Check sheet for the modelled part. Datum: model origin and axes. Units: mm. Face numbers are marked on the shaded views. A direction names the side the tool comes from. Round coordinates to 2 decimals unless told otherwise and drop trailing zeros. Loops run counter-clockwise (first coordinate to the right, second up) from the corner with the lowest first, then second, coordinate; pieces in that order, holes last. Notation, with made-up numbers: M 37.25,40.25 L 75.25,40.25 A18 cw 75.25,64.25 Z; hole C -12.75,-40 d1. An arc over 180 degrees is marked long. Write item = value, one per line. Start each with the question number.
(1) Cross-section at A-A on z = 7. Record the boundary of the cut face in (x, y), plus the area to 3 significant figures.
(2) Scan lines: L1, parallel to Y at x = 0, z = 14.6; L2, parallel to Y at x = 0, z = 10.7; L3, parallel to X at y = 12.5, z = 10.95. Record each from-to range of solid material in increasing order. Write a range as from..to.
(3) Set-up check for the marked faces 1 and 2: record each of +Z, -Z, +X, -X, +Y, -Y from which the full face is reachable in a straight line by a thin tool's end or side.
(4) Mould release check, pull along X, two halves, no side actions. Record for the marked faces 3, 4 and 5: pulls with the +X half, pulls with the -X half, needs draft (parallel to the pull), parting line crosses it, or undercut.
(5) Go/stop test with flat-tipped pins: P1, Ø2, axis at y = 19.5, z = 2.5, coming from the -X side; P2, Ø4, axis at x = 7.5, z = 5.5, coming from the -Y side; P3, Ø1, axis at x = -21, y = 13, coming from the -Z side. Record where each tip stops, or that it passes through.
(6) Cross-section at B-B on x = -11. Record the boundary of the cut face in (y, z).
(7) Cross-section at C-C on y = 5.5. Record the boundary of the cut face in (x, z).
Autodesk Fusion 360 part; units mm, degrees
sketch "Sketch1" plane through (0, 0, 0) normal (0, 0, 1) x (1, 0, 0)
  circle A0 centre (0, 0) radius 30 construction
  circle A1 centre (0, 0) radius 32
  circle A2 centre (0, 0) radius 34
  dimension "d10" = 60
  dimension "d11" = 2
  dimension "d12" = 4
extrude "Extrude1" add sketch "Sketch1" along normal blind 16.6 contours A1 | A2
extrude "Extrude2" cut sketch "Sketch1" along normal blind 12.6 contours A1
sketch "Sketch2" plane through (0, 0, 16.6) normal (0, 0, 1) x (-1, 0, 0)
  circle A0 centre (0, 0) radius 34
  circle A1 centre (0, 0) radius 2.75
  line L0 (0, 0) -> (0, 15) construction
  circle A2 centre (0, 15) radius 3.65
  line L1 (0, 0) -> (-13.0112, 31.4119) construction
  line L2 (0, 0) -> (34, 0) construction
  line L3 (0.4619, 0.1913) -> (-12.5493, 31.6032)
  line L4 (-0.4619, -0.1913) -> (-13.4732, 31.2206)
  line L5 (0.5729, 2.6897) -> (12.5493, 31.6032)
  line L6 (1.4968, 2.307) -> (13.4732, 31.2206)
  line L7 (2.307, 1.4968) -> (31.2206, 13.4732)
  line L8 (2.6897, 0.5729) -> (31.6032, 12.5493)
  line L9 (2.6897, -0.5729) -> (31.6032, -12.5493)
  line L10 (2.307, -1.4968) -> (31.2206, -13.4732)
  line L11 (1.4968, -2.307) -> (13.4732, -31.2206)
  line L12 (0.5729, -2.6897) -> (12.5493, -31.6032)
  line L13 (-0.5729, -2.6897) -> (-12.5493, -31.6032)
  line L14 (-1.4968, -2.307) -> (-13.4732, -31.2206)
  line L15 (-2.307, -1.4968) -> (-31.2206, -13.4732)
  line L16 (-2.6897, -0.5729) -> (-31.6032, -12.5493)
  line L17 (-2.6897, 0.5729) -> (-31.6032, 12.5493)
  line L18 (-2.307, 1.4968) -> (-31.2206, 13.4732)
  circle A3 centre (0, 15) radius 3.15
  line L19 (3.1499, 14.9727) -> (3.1339, 13.1289)
  line L20 (-3.15, 15) -> (-3.15, 13.1561)
  dimension "d35" = 5.5
  dimension "d38" = 15
  dimension "d39" = 7.3
  dimension "d42" = 112.5
  dimension "d43" = 34
  dimension "d50" = 0.5
  dimension "d51" = -0.5
  dimension "d96" = -0.5
extrude "Extrude3" cut sketch "Sketch2" against normal blind 4 contours A1
extrude "Extrude4" cut sketch "Sketch2" against normal blind 4 contours A2 A3 L19 L20 | A2 A3 L19 L20 | A3
extrude "Extrude6" cut sketch "Sketch2" against normal blind 3 contours A0 A1 L7 L8 | A0 A1 L9 L10 | A0 A1 L5 L6 | A0 A1 L11 L12 | A0 A1 L3 L4 | A0 A1 L13 L14 | A0 A1 L17 L18 | A0 A1 L15 L16
extrude "Extrude7" add sketch "Sketch2" against normal blind 0.5 contours A2 A3 L19 L20 | A3 picked at (0.2428, 11.5318)
sketch "Sketch3" plane through (0, 0, 12.6) normal (0, 0, -1) x (1, 0, 0)
  circle A0 centre (0, 15) radius 3.65
  circle A1 centre (0, 0) radius 2.75
  circle A2 centre (0, 0) radius 32
  circle A3 centre (0, 0) radius 25 construction
  line L0 (0, 0) -> (0, 25) construction
  line L1 (0, 25) -> (0, 22) construction
  circle A4 centre (0, 25) radius 1.6
  arc A5 (0, 22) -> (2.1213, 22.8787) centre (0, 25) ccw
  line L2 (2.1213, 22.8787) -> (9.7281, 30.4855)
  line L3 (2.1213, 22.8787) -> (12.8789, 22.8787) construction
  line L4 (-2.1213, 22.8787) -> (-9.7281, 30.4855)
  arc A6 (-2.1213, 22.8787) -> (0, 22) centre (0, 25) ccw
  circle A7 centre (-21.6506, -12.5) radius 1.6
  line L5 (-20.8742, -9.6022) -> (-31.2652, -6.8179)
  arc A8 (-19.0526, -11) -> (-20.8742, -9.6022) centre (-21.6506, -12.5) ccw
  arc A9 (-18.7529, -13.2765) -> (-19.0526, -11) centre (-21.6506, -12.5) ccw
  line L6 (-18.7529, -13.2765) -> (-21.5371, -23.6675)
  circle A10 centre (21.6506, -12.5) radius 1.6
  line L7 (18.7529, -13.2765) -> (21.5371, -23.6675)
  arc A11 (19.0526, -11) -> (18.7529, -13.2765) centre (21.6506, -12.5) ccw
  arc A12 (20.8742, -9.6022) -> (19.0526, -11) centre (21.6506, -12.5) ccw
  line L8 (20.8742, -9.6022) -> (31.2652, -6.8179)
  dimension "d99" = -7
  dimension "d100" = 3
  dimension "d101" = 3.2
  dimension "d102" = 45
  dimension "d104" = 360
extrude "Extrude8" add sketch "Sketch3" along normal blind 3.45 contours A2 A5 L2 L4 A6 | A2 L7 A11 A12 L8 | A2 L5 A8 A9 L6
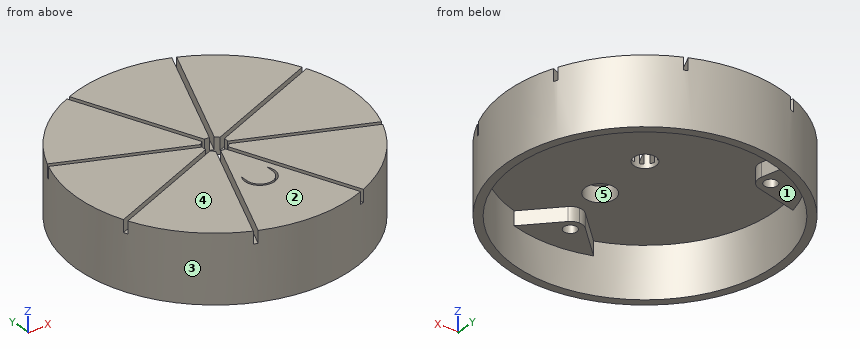
Result:
q1.outline = C 0,0 d68; hole C 0,0 d64
q1.area = 415 mm^2
q2.L1 = -34..-18.65, -11.35..-2.75, 2.75..34
q2.L2 = -34..-26.6, -23.4..-22, 32..34
q2.L3 = -31.62..-23.25, -20.05..-18.65, 18.65..20.05, 23.25..31.62
q3.face_1 = -Z
q3.face_2 = +Z, +X, -X, +Y, -Y
q4.face_3 = parting line crosses it
q4.face_4 = needs draft
q4.face_5 = undercut
q5.P1 = -28.53
q5.P2 = -33.55
q5.P3 = 12.6
q6.outline = M -32.17,0 L -30.05,0 L -30.05,12.6 L 30.05,12.6 L 30.05,0 L 32.17,0 L 32.17,16.6 L 27.86,16.6 L 27.86,13.6 L 25.25,13.6 L 25.25,16.6 L 5.1,16.6 L 5.1,13.6 L 4.02,13.6 L 4.02,16.6 L -4.02,16.6 L -4.02,13.6 L -5.1,13.6 L -5.1,16.6 L -25.25,16.6 L -25.25,13.6 L -27.86,13.6 L -27.86,16.6 L -32.17,16.6 Z
q7.outline = M -33.55,0 L -31.52,0 L -31.52,12.6 L 31.52,12.6 L 31.52,0 L 33.55,0 L 33.55,16.6 L 14.58,16.6 L 14.58,13.6 L 11.97,13.6 L 11.97,16.6 L 2.82,16.6 L 2.82,13.6 L 1.74,13.6 L 1.74,16.6 L -1.74,16.6 L -1.74,13.6 L -2.82,13.6 L -2.82,16.6 L -11.97,16.6 L -11.97,13.6 L -14.58,13.6 L -14.58,16.6 L -33.55,16.6 Z
